Read the model definition and answer for the solid it produces. Units are mm, in the model's axes. Face numbers are marked on the shaded views. A direction names the side the tool comes from. Coordinates: 2 decimals unless noted, no trailing zeros. Order: outer loops, then holes, each group sorted by start corner. A loop starts at its lowest first (then second) coordinate and runs counter-clockwise, first axis right, second up. Notation, with made-up numbers: (44, 67) - (84, 67) arc R28 cw to (84, 106) - close; hole circle Ø9 at (16, 80). An arc over 180 degrees is marked (long way). Write item = value, one per line.
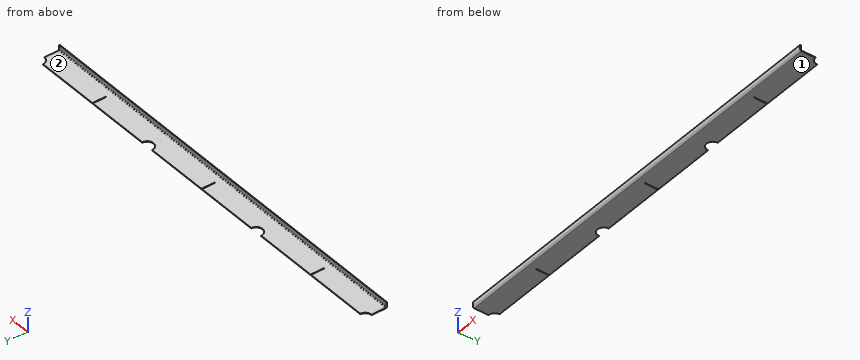
Autodesk Inventor part; units mm, degrees
ref_plane "YZ Plane" through (0, 0, 0) normal (1, 0, 0) x (0, 1, 0)
ref_plane "XZ Plane" through (0, 0, 0) normal (0, 1, 0) x (-1, 0, 0)
ref_plane "XY Plane" through (0, 0, 0) normal (0, 0, 1) x (1, 0, 0)
sketch "Sketch1" plane through (0, 0, 0) normal (0, 0, 1) x (1, 0, 0)
  line L0 (-750, 77.7055) -> (750, 77.7055)
  line L1 (750, 77.7055) -> (750, 0)
  line L2 (750, 0) -> (-750, 0)
  line L3 (-750, 0) -> (-750, 77.7055)
  point P0 (0, 0)
  point P1 (0, 0)
  dimension "d0" = 1500
  dimension "d1" = 77.7056
extrude "Plate1" add sketch "Sketch1" along normal blind 2
sketch "Sketch2" plane through (750, 2, 0) normal (0, -1, 0) x (1, 0, 0)
  line L0 (-1500, 0) -> (0, 0)
  line L1 (0, 0) -> (0, 20)
  line L2 (0, 20) -> (-1500, 20)
  line L3 (-1500, 20) -> (-1500, 0)
edge flange "Flange1" height 20 angle 90 thickness 2 bend radius 2.75 thickness toward (0, -1, 0) relief round relief width 2 relief depth 1 edges at (0, 0, 2) wall of the first edge with corners at (-750, 2, 0) (750, 2, 0) (750, 2, 20) (-750, 2, 20)
bend "Bend1"
corner "Corner1"
sketch "Sketch5" plane through (0, 0, 0) normal (0, 0, -1) x (-1, 0, 0)
  line L0 (750, 77.7055) -> (-750, 77.7055)
  line L1 (-1, 30) -> (-1, 77.7055)
  line L2 (750, 0) -> (-750, 0)
  line L3 (-1, 30) -> (1, 30)
  line L4 (1, 30) -> (1, 77.7055)
  point P0 (0, 0)
  point P1 (0, 30)
  point P2 (0, 0)
  dimension "d27" = 2
  dimension "d28" = 30
extrude "Extrusion1" cut sketch "Sketch5" against normal through all
pattern_linear "Rectangular Pattern1" count 3 spacing 500 along (1, 0, 0) of "Extrusion1" first direction both ways yes
sketch "Sketch6" plane through (0, 0, 0) normal (0, 0, -1) x (-1, 0, 0)
  line L0 (-750, 77.7055) -> (-750, 4.75)
  circle A0 centre (-750, 77.7055) radius 22.5
  line L1 (-750, 77.7055) -> (750, 77.7055)
  line L2 (-1, 77.7055) -> (-1, 30)
  line L3 (-499, 77.7055) -> (-499, 30)
  line L4 (-1, 30) -> (-499, 30) construction
  circle A1 centre (-250, 77.7055) radius 22.5
  point P0 (0, 0)
  point P1 (-727.5, 77.7055)
  point P2 (-750, 55.2055)
  point P3 (-250, 30)
  dimension "d24" = 45
extrude "Extrusion2" cut sketch "Sketch6" along normal mid plane 30 contours L1 A0 L0 | A1 L1 | L1 A1 picked at (-748.3311, 62.8935)
mirror "Mirror1" about plane through (0, 0, 0) normal (1, 0, 0) of "Extrusion2"
sketch "Sketch7" plane through (0, 0, 2) normal (0, 0, 1) x (1, 0, 0)
  arc A0 (-750, 55.2055) -> (-727.5, 77.7055) centre (-750, 77.7055) ccw
  line L0 (-750, 4.75) -> (-750, 55.2055)
  line L1 (-750, 4.75) -> (750, 4.75)
  line L2 (750, 55.2055) -> (750, 4.75)
  arc A1 (727.5, 77.7055) -> (750, 55.2055) centre (750, 77.7055) ccw
  line L3 (501, 77.7055) -> (727.5, 77.7055)
  line L4 (501, 77.7055) -> (501, 30)
  line L5 (501, 30) -> (499, 30)
  line L6 (499, 30) -> (499, 77.7055)
  line L7 (1, 77.7055) -> (227.5, 77.7055)
  line L8 (1, 77.7055) -> (1, 30)
  line L9 (1, 30) -> (-1, 30)
  line L10 (-1, 30) -> (-1, 77.7055)
  line L11 (-499, 77.7055) -> (-272.5, 77.7055)
  line L12 (-499, 77.7055) -> (-499, 30)
  line L13 (-499, 30) -> (-501, 30)
  line L14 (-501, 30) -> (-501, 77.7055)
  line L15 (-727.5, 77.7055) -> (-501, 77.7055)
  line L16 (750, 4.75) -> (-750, 4.75)
  line L17 (650, 4.75) -> (650, 77.7055) construction
  line L18 (-750, 4.75) -> (750, 4.75)
  line L19 (646, 37.7637) -> (650, 44.6919)
  line L20 (650, 44.6919) -> (654, 37.7637)
  line L21 (654, 37.7637) -> (646, 37.7637)
  line L22 (650, 44.6919) -> (650, 37.7637) construction
  line L23 (626, 37.7637) -> (630, 44.6919)
  line L24 (630, 44.6919) -> (634, 37.7637)
  line L25 (634, 37.7637) -> (626, 37.7637)
  line L26 (630, 44.6919) -> (630, 37.7637) construction
  line L27 (272.5, 77.7055) -> (499, 77.7055)
  arc A2 (227.5, 77.7055) -> (272.5, 77.7055) centre (250, 77.7055) ccw
  line L28 (-227.5, 77.7055) -> (-1, 77.7055)
  arc A3 (-272.5, 77.7055) -> (-227.5, 77.7055) centre (-250, 77.7055) ccw
  point P0 (0, 0)
  point P1 (650, 41.2278)
  point P2 (630, 41.2278)
  dimension "d29" = 100
  dimension "d30" = 8
  dimension "d31" = 8
  dimension "d32" = 20
extrude "Extrusion3" [suppressed]
mirror "Mirror2" [suppressed]
sketch "Sketch8" plane through (0, 0, 2) normal (0, 0, 1) x (1, 0, 0)
  line L0 (496, 72.7055) -> (496, 60.7055) construction
  line L1 (496, 60.7055) -> (296, 60.7055) construction
  line L2 (296, 60.7055) -> (296, 72.7055) construction
  line L3 (296, 72.7055) -> (496, 72.7055) construction
  line L4 (501, 77.7055) -> (727.5, 77.7055)
  line L5 (272.5, 77.7055) -> (499, 77.7055)
  point P0 (0, 0)
  dimension "d35" = 200
  dimension "d36" = 12
  dimension "d39" = 3
  dimension "d40" = 5
mark "Mark1"
equation "\"d1\" = Стрингер_6"
equation "\"d27\" = d18"
equation "\"d2\" = Thickness"
equation "\"d3\" = BendReliefWidth"
equation "\"d4\" = BendReliefDepth"
equation "\"d5\" = MinimumRemnant"
equation "\"d6\" = TransitionRadius"
equation "\"d9\" = BendRadius"
equation "\"d10\" = CornerReliefSize"
equation "\"d11\" = GapSize"
equation "\"d12\" = JacobiRadiusSize"
equation "\"BendReliefWidth\" = Thickness"
equation "\"BendReliefDepth\" = 0.5 * Thickness"
equation "\"CornerReliefSize\" = 4 * Thickness"
equation "\"MinimumRemnant\" = 2 * Thickness"
equation "\"TransitionRadius\" = BendRadius"
equation "\"JacobiRadiusSize\" = BendRadius"
equation "\"GapSize\" = Thickness"
equation "\"d18\" = Thickness"
properties part number "MSC 066 stringer board ####" material "Stainless Steel"
1) Straight lines are drawn through the part: line 1 along X through (y, z) = (31, 1.5); line 2 along Z through (x, y) = (-682.5, 29); line 3 along Y through (x, z) = (-243.5, 4.5). For each, find the intervals that lie inside material, in ascending order. Write a range as from..to.
Returned:
line_1 = -750..-501, -499..-1, 1..499, 501..750
line_2 = 0..2
line_3 = 0.01..2.01
2) Flat-ended cylindrical pins translate along their axes: pin 1 Ø1 at (y, z) = (63.5, 1) entering from -X; pin 2 Ø12 at (x, z) = (539, 16.5) entering from +Y; pin 3 Ø5 at (x, y) = (222, 39) entering from +Z. Find the tip coordinate at first contact, or state that the pin passes through.
Returned:
pin_1 = -732.97
pin_2 = 2
pin_3 = 2
3) The part is cut by section C-C (x = -250). Determine the outline of the cut face in (y, z), and give its area (3 significant figures).
Returned:
outline = (0, 4.75) arc R4.75 ccw to (4.75, 0) - (55.21, 0) - (55.21, 2) - (4.75, 2) arc R2.75 cw to (2, 4.75) - (2, 20) - (0, 20) - close
area = 143 mm^2
4) The part is cut by section A-A (x = -580.5). Determine the outline of the cut face in (y, z), and give its area (3 significant figures).
Returned:
outline = (0, 4.75) arc R4.75 ccw to (4.75, 0) - (77.71, 0) - (77.71, 2) - (4.75, 2) arc R2.75 cw to (2, 4.75) - (2, 20) - (0, 20) - close
area = 188 mm^2
5) For the marked faces 1 and 2, determine the directions among +Z, -Z, +X, -X, +Y, -Y from which every point of the face is accessible in a straight line to the end or side of a thin tool.
Returned:
face_1 = -Z, +X, -X, +Y, -Y
face_2 = +Z, +X, -X, +Y
6) The part is cut by section B-B (z = 12.5). Determine the outline of the cut face in (x, y).
Returned:
outline = (-750, 0) - (750, 0) - (750, 2) - (-750, 2) - close
